from build123d import *


with BuildPart() as part:
    # Sketch1 → Revolve1 (revolve)
    with BuildSketch(Plane.XY):
        with BuildLine():
            Line((0, 1127), (0, 1122))
            ThreePointArc((0, 1122), (86.267027305, 1086.267027305), (122, 1000))
            Line((122, 1000), (122, 950))
            Line((122, 950), (124.5, 950))
            Line((124.5, 950), (124.5, 975))
            Line((124.5, 975), (127, 975))
            Line((127, 975), (127, 1000))
            ThreePointArc((127, 1000), (89.802561211, 1089.802561211), (0, 1127))
        make_face()
    revolve(axis=Axis((0, 1000, 0), (0, -1, 0)))


solid = part.part
Could you check a few things on this model? Use its own coordinates, in mm. A direction names the side the tool comes from. Coordinates: 2 decimals unless noted, no trailing zeros. Order: outer loops, then holes, each group sorted by start corner. A loop starts at its lowest first (then second) coordinate and runs counter-clockwise, first axis right, second up.
Q1. Will these pins go through, and if not, where does the flat tip stop? pin 1 (1 mm diameter, centred on x = -10, z = -88.5, fed in from +Y); pin 2 (6 mm diameter, centred on x = -45, z = -66.5, fed in from +Y); pin 3 (6 mm diameter, centred on x = 56.5, z = -7, fed in from -Y).
Q2. Suppose I cut it at D-D on z = 0. Please give me the cut outline in (x, y), and give its area (3 significant figures).
Q3. Please list where these lines run through material, in increasing order: L1, parallel to Z at x = 0, y = 964; L2, parallel to Z at x = 0, y = 981; L3, parallel to X at y = 1044, z = 78.
Q4. Suppose I cut it at B-B on z = -25.5. Please give me the cut outline in (x, y).
Q5. Suppose I cut it at A-A on x = 0. Please give me the cut outline in (y, z), and give its area (3 significant figures).
Q6. Which directions (+Z, -Z, +X, -X, +Y, -Y) give clear straight access to the entire face, cutting with the end or side of a thin tool? Please do faces 1 (the cylindrical face through (57.449, 962.675, -110.453)), 2 (the flat face through (-82, 950, -92)).
Q7. Suppose I cut it at C-C on y = 1051.5. Please give me the cut outline in (x, z).
Q8. Thinking about a two-plate mould opening in X: for faces 3 (the cylindrical face through (-96.815, 974.65, -74.235)), 4 (the cylindrical face through (-27.53, 987.68, -123.98)), 5 (the flat face through (-84, 975, -93)), which applies, released by +X, released by -X, zero draft, split by the parting line, or undercut?
Answer:
1. pin 1: stops at y = 1091.03
1. pin 2: stops at y = 1100.77
1. pin 3: stops at y = 1106.26
2. outline: (-127, 975) - (-124.5, 975) - (-124.5, 950) - (-122, 950) - (-122, 1000) arc R122 cw to (122, 1000) - (122, 950) - (124.5, 950) - (124.5, 975) - (127, 975) - (127, 1000) arc R127 ccw to (-127, 1000) - close
2. area: 2,330 mm2
3. L1: z = -124.5 to -122, 122 to 124.5
3. L2: z = -127 to -122, 122 to 127
3. L3: x = -90.05 to -82.85, 82.85 to 90.05
4. outline: (-124.41, 975) - (-121.86, 975) - (-121.86, 950) - (-119.31, 950) - (-119.31, 1000) arc R119.31 cw to (119.31, 1000) - (119.31, 950) - (121.86, 950) - (121.86, 975) - (124.41, 975) - (124.41, 1000) arc R124.41 ccw to (-124.41, 1000) - close
5. outline: (950, -124.5) - (975, -124.5) - (975, -127) - (1000, -127) arc R127 ccw to (1000, 127) - (975, 127) - (975, 124.5) - (950, 124.5) - (950, 122) - (1000, 122) arc R122 cw to (1000, -122) - (950, -122) - close
5. area: 2,330 mm2
6. face 1: -Y
6. face 2: +Z, -Z, +X, -X, -Y
7. outline: circle Ø232.18 at (0, 0); hole circle Ø221.19 at (0, 0)
8. face 3: undercut
8. face 4: split by the parting line
8. face 5: zero draft
